Autodesk Inventor part; units mm, degrees
ref_plane "YZ Plane" through (0, 0, 0) normal (1, 0, 0) x (0, 1, 0)
ref_plane "XZ Plane" through (0, 0, 0) normal (0, 1, 0) x (-1, 0, 0)
ref_plane "XY Plane" through (0, 0, 0) normal (0, 0, 1) x (1, 0, 0)
sketch "Эскиз1" plane through (0, 0, 0) normal (0, 1, 0) x (-1, 0, 0)
  line L0 (7.05, -7.05) -> (-7.05, -7.05)
  line L1 (-7.05, -7.05) -> (-7.05, 7.05)
  line L2 (-7.05, 7.05) -> (7.05, 7.05)
  line L3 (7.05, 7.05) -> (7.05, -7.05)
  line L4 (7.05, -7.05) -> (-7.05, 7.05) construction
  line L5 (-7.05, -7.05) -> (7.05, 7.05) construction
  line L6 (-10, -10) -> (10, -10)
  line L7 (10, -10) -> (10, 10)
  line L8 (10, 10) -> (-10, 10)
  line L9 (-10, 10) -> (-10, -10)
  line L10 (-10, -10) -> (10, 10) construction
  line L11 (10, -10) -> (-10, 10) construction
  point P0 (0, 0)
  dimension "d0" = 14.1
  dimension "d1" = 14.1
  dimension "d2" = 20
  dimension "d3" = 20
extrude "Выдавливание1" add sketch "Эскиз1" along normal blind 9
sketch "Эскиз2" plane through (-10, 0, 10) normal (0, 0, 1) x (1, 0, 0)
  line L0 (0, 0) -> (0, 9)
  line L1 (20, 9) -> (0, 9)
  line L2 (0, 0) -> (20, 9)
  line L3 (0, 9) -> (20, 0)
  line L4 (0, 4.5) -> (20, 4.5)
  line L5 (20, 0) -> (0, 0)
  line L6 (20, 4.5) -> (0, 0)
  line L7 (0, 4.5) -> (20, 0)
  line L8 (10, 2.25) -> (2, 2.25)
  line L9 (2, 2.25) -> (18, 2.25)
  circle A0 centre (2, 2.25) radius 1
  circle A1 centre (18, 2.25) radius 1
  circle A2 centre (10, 6.5217) radius 1
  circle A3 centre (10, 6.5217) radius 2
  point P0 (10, 0)
  dimension "d6" = 8
  dimension "d7" = 16
  dimension "d8" = 2
  dimension "d9" = 2
  dimension "d10" = 2
  dimension "d11" = 4
sketch "Эскиз3" plane through (-10, 0, 10) normal (0, 0, 1) x (1, 0, 0)
  circle A0 centre (10, 6.5383) radius 2
  point P0 (10, 0)
  dimension "d12" = 4
extrude "Выдавливание2" cut sketch "Эскиз2" against normal blind 25 contours A1 | A0 | A2
sketch "Эскиз4" plane through (10, 0, -10) normal (0, 0, -1) x (-1, 0, 0)
  circle A0 centre (10, 6.5217) radius 1
  circle A1 centre (10, 6.5217) radius 2
  point P0 (10, 0)
  dimension "d15" = 4
extrude "Выдавливание3" cut sketch "Эскиз3" against normal blind 2
extrude "Выдавливание4" cut sketch "Эскиз4" against normal blind 2
fillet "Сопряжение1" radius 1 4 edges at (-10, 4.5, 10) (10, 4.5, 10) (10, 4.5, -10) (-10, 4.5, -10)
Design review of the part built by this model. Coordinates are the model's own, in mm. A direction names the side the tool comes from. Round coordinates to 2 decimals unless told otherwise and drop trailing zeros. Write each loop counter-clockwise with the first axis right and the second up, starting at its lowest first coordinate (ties: lowest second). Pieces come first, ordered by that corner, then holes.
Item 1: The part is to be moulded in two halves that separate along X. For faces 1 (the cylindrical face through (-9.715, 4.563, 9.699)), 2 (the cylindrical face through (-0.13, 7.513, -7.518)), 3 (the cylindrical face through (9.715, 4.563, -9.699)), 4 (the flat face through (9, 9, 0)), say which applies: +X half, -X half, draft (parallel to the pull), parting line (faces both ways), or undercut.
Item 2: We need section D-D on x = 8. Write out the cut boundary in (y, z), and give its area (3 significant figures).
Item 3: For faces 5 (the cylindrical face through (-0.434, 4.586, 9.014)), 6 (the flat face through (0, 4, 7.05)), 7 (the flat face through (10, 4, 0)), list the 3-axis set-ups (+Z, -Z, +X, -X, +Y, -Y) from which the entire face can be reached by the end or side of a thin tool; tool diameter is ignored.
Item 4: We need section C-C on y = 1. Write out the cut boundary in (x, z).
Item 5: For probe 1 along Y at (x, z) = (8, 2.5); probe 2 along X at (y, z) = (6, -4.75), list the stretches that pass through material, from the lowest coordinate up.
Item 6: Clearance check with flat-ended pins moving along their axes: pin 1 Ø1.2 at (x, y) = (1, 6.5) entering from -Z; pin 2 Ø3 at (x, y) = (0, 6.52) entering from +Z; pin 3 Ø1.6 at (x, y) = (0, 6.52) entering from -Z. State where each tip first meets the part, or that it passes through.
Item 7: We need section A-A on z = 0.25. Write out the cut boundary in (x, y).
Item 8: We need section B-B on x = 0. Write out the cut boundary in (y, z), and give its area (3 significant figures).
Returned:
1. face 1: -X half
1. face 2: undercut
1. face 3: +X half
1. face 4: draft
2. outline: (0, -10) - (1.25, -10) - (1.25, 10) - (0, 10) - close; (3.25, -10) - (9, -10) - (9, 10) - (3.25, 10) - close
2. area: 140 mm2
3. face 5: +Z
3. face 6: +Y, -Y
3. face 7: +Z, -Z, +X, +Y, -Y
4. outline: (-10, -9) arc R1 ccw to (-9, -10) - (9, -10) arc R1 ccw to (10, -9) - (10, 9) arc R1 ccw to (9, 10) - (-9, 10) arc R1 ccw to (-10, 9) - close; hole (-7.05, -7.05) - (7.05, -7.05) - (7.05, 7.05) - (-7.05, 7.05) - close
5. probe 1: y = 0 to 1.25, 3.25 to 9
5. probe 2: x = -10 to -7.05, 7.05 to 10
6. pin 1: stops at z = -8
6. pin 2: stops at z = 8
6. pin 3: passes through
7. outline: (-10, 0) - (-7.05, 0) - (-7.05, 1.94) arc R1 cw (long way) to (-7.05, 2.56) - (-7.05, 9) - (-10, 9) - close; (7.05, 0) - (10, 0) - (10, 9) - (7.05, 9) - (7.05, 2.56) arc R1 cw (long way) to (7.05, 1.94) - close
8. outline: (0, -10) - (4.52, -10) - (4.52, -8) - (5.52, -8) - (5.52, -7.05) - (0, -7.05) - close; (0, 7.05) - (5.52, 7.05) - (5.52, 8) - (4.54, 8) - (4.54, 10) - (0, 10) - close; (7.52, -8) - (8.52, -8) - (8.52, -10) - (9, -10) - (9, -7.05) - (7.52, -7.05) - close; (7.52, 7.05) - (9, 7.05) - (9, 10) - (8.54, 10) - (8.54, 8) - (7.52, 8) - close
8. area: 33.3 mm2
